Source: three-view drawing plus pictorial views. Frame: mm from the lowest corner of the part. Coordinates: 2 decimals unless noted, no trailing zeros. Loops run counter-clockwise (first coordinate to the right, second up) from the corner with the lowest first, then second, coordinate; pieces in that order, holes last. Notation, with made-up numbers: (23, 69) - (80, 69) arc R13 cw to (80, 85) - close; hole circle Ø10 at (-11, 31). An arc over 180 degrees is marked (long way). Answer as CSV lines item,"result". Start each with the question number.
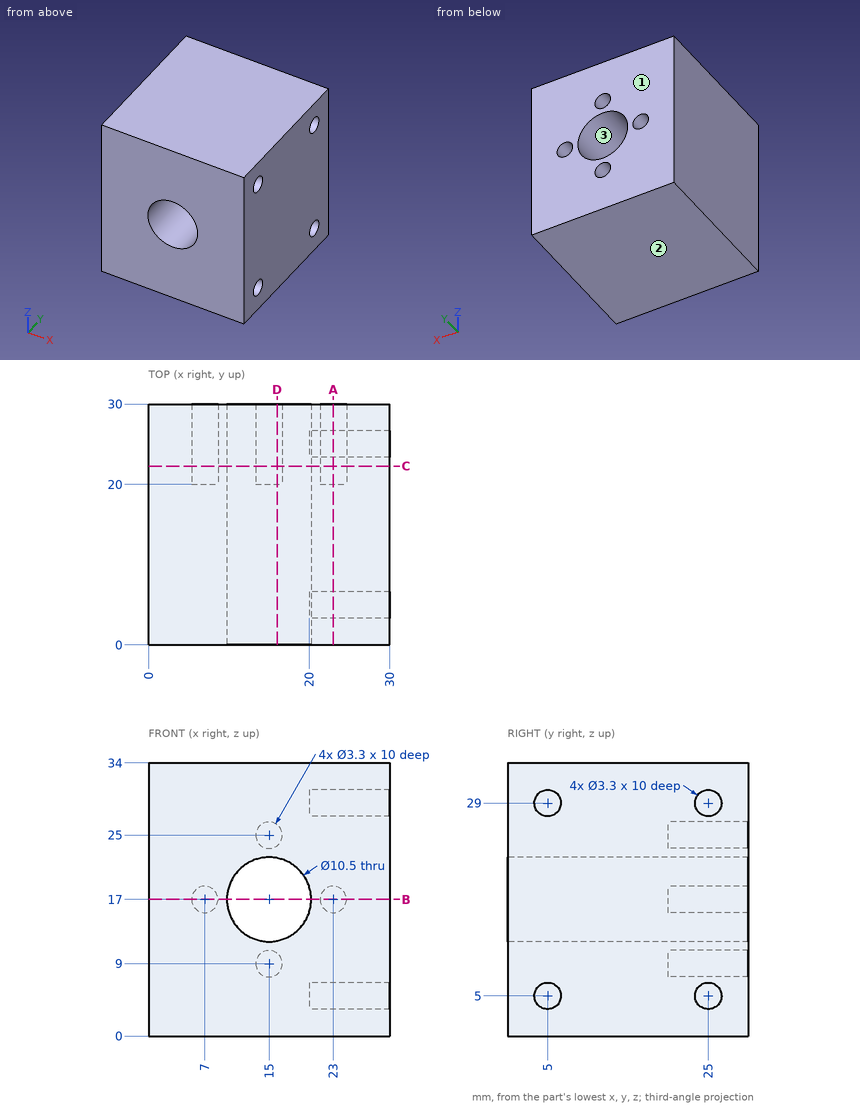
Item 1: Section query B-B, the plane z = 17. Output: boundary loops of the cut face in (x, y), and give its area (3 significant figures).
Item 2: Material intervals for probe 1 along Y at (x, z) = (26.5, 5); probe 2 along Z at (x, y) = (23, 28.25); probe 3 along Z at (x, y) = (15, 6.5), sorted ascending.
Item 3: Contact query for flat-ended pins moving along their axis: P1, Ø3.5, axis at y = 6, z = 28.5, coming from the +X side; P2, Ø1, axis at x = 23, z = 17.5, coming from the +Y side; P3, Ø3, axis at y = 5, z = 29, coming from the +X side. Output: stop coordinate, or through.
Item 4: Section query C-C, the plane y = 22.25. Output: boundary loops of the cut face in (x, z), and give its area (3 significant figures).
Item 5: Draft query along Z for the marked faces 1, 2 and 3. Return one class per face: pulls with the +Z half, pulls with the -Z half, needs draft (parallel to the pull), parting line crosses it, or undercut.
Item 6: Section query A-A, the plane x = 23. Output: boundary loops of the cut face in (y, z).
Item 7: Section query D-D, the plane x = 16. Output: boundary loops of the cut face in (y, z), and give its area (3 significant figures).
Response values:
1,outline,"(0, 0) - (9.75, 0) - (9.75, 30) - (8.65, 30) - (8.65, 20) - (5.35, 20) - (5.35, 30) - (0, 30) - close; (20.25, 0) - (30, 0) - (30, 30) - (24.65, 30) - (24.65, 20) - (21.35, 20) - (21.35, 30) - (20.25, 30) - close"
1,area,"519 mm²"
2,probe 1,"y = 0 to 3.35, 6.65 to 23.35, 26.65 to 30"
2,probe 2,"z = 0 to 15.35, 18.65 to 34"
2,probe 3,"z = 0 to 11.75, 22.25 to 34"
3,P1,"stops at x = 30"
3,P2,"stops at y = 20"
3,P3,"stops at x = 20"
4,outline,"(0, 0) - (30, 0) - (30, 34) - (0, 34) - close; hole circle Ø3.3 at (7, 17); hole circle Ø10.5 at (15, 17); hole circle Ø3.3 at (15, 9); hole circle Ø3.3 at (15, 25); hole circle Ø3.3 at (23, 17)"
4,area,"899 mm²"
5,face 1,"needs draft"
5,face 2,"pulls with the -Z half"
5,face 3,"undercut"
6,outline,"(0, 0) - (30, 0) - (30, 15.35) - (20, 15.35) - (20, 18.65) - (30, 18.65) - (30, 34) - (0, 34) - close; hole circle Ø3.3 at (5, 5); hole circle Ø3.3 at (5, 29); hole circle Ø3.3 at (25, 5); hole circle Ø3.3 at (25, 29)"
7,outline,"(0, 0) - (30, 0) - (30, 7.69) - (20, 7.69) - (20, 10.31) - (30, 10.31) - (30, 11.85) - (0, 11.85) - close; (0, 22.15) - (30, 22.15) - (30, 23.69) - (20, 23.69) - (20, 26.31) - (30, 26.31) - (30, 34) - (0, 34) - close"
7,area,"658 mm²"
